Source: three-view drawing plus pictorial views. Frame: mm from the lowest corner of the part. Give positions to 0.01 mm unless a question says otherwise; leave off trailing zeros. Loops run counter-clockwise (first coordinate to the right, second up) from the corner with the lowest first, then second, coordinate; pieces in that order, holes last. Notation, with made-up numbers: (85, 16.25) -> (92, 16.25) arc R16 cw to (92, 34.25) -> close; hole circle Ø2 at (60.25, -38.5). An arc over 180 degrees is marked (long way). Answer in a Markdown table with one row per item. Add a question column.
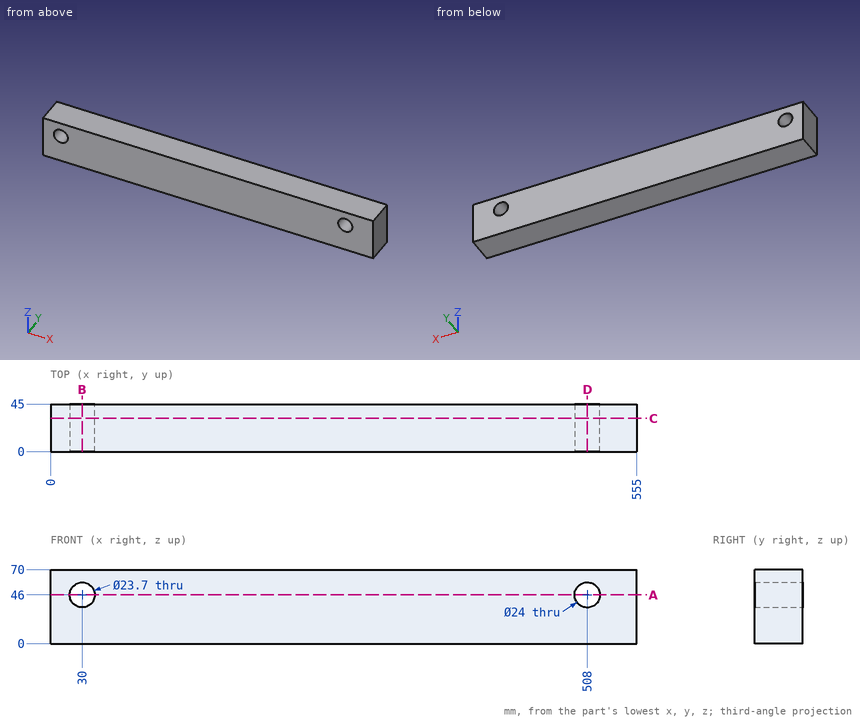
(1) Cut plane C-C on y = 31.5. Return the cut outline in (x, z).
(2) Cut plane A-A on z = 46. Return the cut outline in (x, y).
(3) Material intervals for line 1 along X through (y, z) = (39.5, 46.5); line 2 along Z through (x, y) = (508, 10); line 3 along Z through (x, y) = (30, 19), sorted ascending. Write a range as from..to.
(4) Cut plane B-B on x = 30. Return the cut outline in (y, z), then the cut area to 3 significant figures.
(5) Cut plane D-D on x = 508. Return the cut outline in (y, z).
Answer list:
| question | item | result |
|---|---|---|
| 1 | outline | (0, 0) -> (555, 0) -> (555, 70) -> (0, 70) -> close; hole circle Ø23.7 at (30, 46); hole circle Ø24 at (508, 46) |
| 2 | outline | (0, 0) -> (18.15, 0) -> (18.15, 45) -> (0, 45) -> close; (41.85, 0) -> (496, 0) -> (496, 45) -> (41.85, 45) -> close; (520, 0) -> (555, 0) -> (555, 45) -> (520, 45) -> close |
| 3 | line 1 | x = 0..18.16, 41.84..496.01, 519.99..555 |
| 3 | line 2 | z = 0..34, 58..70 |
| 3 | line 3 | z = 0..34.15, 57.85..70 |
| 4 | outline | (0, 0) -> (45, 0) -> (45, 34.15) -> (0, 34.15) -> close; (0, 57.85) -> (45, 57.85) -> (45, 70) -> (0, 70) -> close |
| 4 | area | 2,080 mm² |
| 5 | outline | (0, 0) -> (45, 0) -> (45, 34) -> (0, 34) -> close; (0, 58) -> (45, 58) -> (45, 70) -> (0, 70) -> close |
